```python
from build123d import *

# Parameters (mm, degrees)
SKIZZE1_R                       = 1.6
AUFSATZ_LINEAR_AUSTRAGEN1_DEPTH = 5


with BuildPart() as part:
    # Skizze1 → Aufsatz-Linear austragen1 (new body)
    with BuildSketch(Plane.XY):
        Polygon((5, 10), (5, 20), (0, 20), (0, 30), (5, 30), (5, 40), (0, 40), (0, 50), (5, 50), (5, 60), (0, 60), (0, 70), (5, 70), (5, 80), (0, 80), (0, 90), (5, 90), (5, 100), (0, 100), (0, 110), (5, 110), (5, 120), (0, 120), (0, 130), (5, 130), (5, 140), (0, 140), (0, 150), (5, 150), (5, 160), (0, 160), (0, 170), (5, 170), (5, 180), (0, 180), (0, 190), (5, 190), (5, 200), (0, 200), (0, 210), (5, 210), (5, 220), (35, 250), (45, 250), (45, 255), (55, 255), (55, 250), (65, 250), (65, 255), (75, 255), (75, 250), (85, 250), (85, 255), (95, 255), (95, 250), (105, 250), (105, 255), (115, 255), (115, 250), (125, 250), (125, 255), (135, 255), (135, 250), (145, 250), (145, 255), (155, 255), (155, 250), (165, 250), (165, 255), (175, 255), (175, 250), (185, 250), (185, 255), (195, 255), (195, 250), (205, 250), (205, 255), (215, 255), (215, 250), (225, 250), (225, 255), (235, 255), (235, 250), (245, 250), (245, 255), (255, 255), (255, 250), (265, 250), (265, 255), (275, 255), (275, 250), (305, 220), (305, 210), (310, 210), (310, 200), (305, 200), (305, 190), (310, 190), (310, 180), (305, 180), (305, 170), (310, 170), (310, 160), (305, 160), (305, 150), (310, 150), (310, 140), (305, 140), (305, 130), (310, 130), (310, 120), (305, 120), (305, 110), (310, 110), (310, 100), (305, 100), (305, 90), (310, 90), (310, 80), (305, 80), (305, 70), (310, 70), (310, 60), (305, 60), (305, 50), (310, 50), (310, 40), (305, 40), (305, 30), (310, 30), (310, 20), (305, 20), (305, 10), (310, 10), (310, 0), (305, 0), (5, 0), (0, 0), (0, 10), align=None)
        with Locations((290, 214.999999999)):
            Circle(SKIZZE1_R, mode=Mode.SUBTRACT)
        with Locations((280, 214.999999999)):
            Circle(SKIZZE1_R, mode=Mode.SUBTRACT)
        with Locations((20, 215)):
            Circle(SKIZZE1_R, mode=Mode.SUBTRACT)
        with Locations((30, 215)):
            Circle(SKIZZE1_R, mode=Mode.SUBTRACT)
        Polygon((275, 188.971165398), (245, 218.971165398), (65, 218.971165398), (35, 188.971165398), (35, 78.971165398), (275, 78.971165398), align=None, mode=Mode.SUBTRACT)
    extrude(amount=AUFSATZ_LINEAR_AUSTRAGEN1_DEPTH)


solid = part.part
```
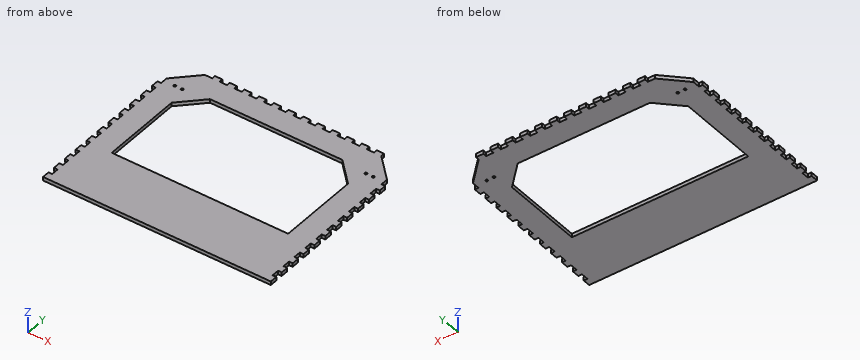
Verification items for the finished model (mm, model axes). Round coordinates to 2 decimals unless told otherwise and drop trailing zeros. Loops run counter-clockwise (first coordinate to the right, second up) from the corner with the lowest first, then second, coordinate; pieces in that order, holes last. Notation, with made-up numbers: (39, 53.25) -> (75, 53.25) arc R16 cw to (75, 68.25) -> close; hole circle Ø7 at (68, -34.75). An arc over 180 degrees is marked (long way). Answer as a JSON object with one key per item and string values.
Q1. Go/stop test with flat-tipped pins: P1, Ø1.5, axis at x = 3.5, z = 3, coming from the +Y side; P2, Ø2.5, axis at x = 60.5, z = 3, coming from the +Y side; P3, Ø1.5, axis at y = 253.5, z = 3, coming from the -X side. Record where each tip stops, or that it passes through.
Data:
{"P1": "stops at y = 210", "P2": "stops at y = 250", "P3": "stops at x = 45"}
Q2. Scan lines: line 1 (Y direction, x = 213, z = 0.85); line 2 (Y direction, x = 30, z = 1.6); line 3 (X direction, y = 182, z = 4.75). Record each from-to range of solid material in increasing order. Write a range as from..to.
Data:
{"line 1": "y = 0..78.97, 218.97..255", "line 2": "y = 0..213.4, 216.6..245", "line 3": "x = 0..35, 275..310"}
Q3. Section check C-C (z = 0.75). State how many separate pieces and enclosed holes the cut face has, then the cut area to 3 significant figures.
Data:
{"separate pieces": "1", "enclosed holes": "5", "area": "43,100 mm2"}
Q4. Section check B-B (x = 259). Record the boundary of the cut face in (y, z), then the cut area to 3 significant figures.
Data:
{"outline": "(0, 0) -> (78.97, 0) -> (78.97, 5) -> (0, 5) -> close; (204.97, 0) -> (250, 0) -> (250, 5) -> (204.97, 5) -> close", "area": "620 mm2"}
Q5. Section check A-A (x = 88.5). Record the boundary of the cut face in (y, z), then the cut area to 3 significant figures.
Data:
{"outline": "(0, 0) -> (78.97, 0) -> (78.97, 5) -> (0, 5) -> close; (218.97, 0) -> (255, 0) -> (255, 5) -> (218.97, 5) -> close", "area": "575 mm2"}
